Source: CAD feature listing. Evaluate the final solid. Frame: model axes, mm. Face numbers are marked on the shaded views. A direction names the side the tool comes from. Give positions to 0.01 mm unless a question says otherwise; leave off trailing zeros. Loops run counter-clockwise (first coordinate to the right, second up) from the corner with the lowest first, then second, coordinate; pieces in that order, holes last. Notation, with made-up numbers: (75, 40.5) - (82, 40.5) arc R30 ccw to (82, 77.5) - close; hole circle Ø10 at (78.25, 2). An arc over 180 degrees is marked (long way). Write each question's results on one line, items separated by ' | '. Start each with the question number.
(1) Contact query for flat-ended pins moving along their axis: pin 1 (2 mm diameter, centred on x = -11, z = -7.5, fed in from -Y); pin 2 (1.2 mm diameter, centred on y = -0.5, z = 0.5, fed in from -X); pin 3 (3 mm diameter, centred on x = 10.5, z = -3.5, fed in from +Y). Output: stop coordinate, or through.
(2) Material intervals for line 1 along Z through (x, y) = (-11.75, 0.3); line 2 along Z through (x, y) = (-8.25, -0.75); line 3 along X through (y, z) = (-0.1, -2.5), sorted ascending. Write a range as [from, to].
(3) Cut plane A-A on y = -0.8. Return the cut outline in (x, z).
(4) Reachability of the marked faces 1 and 2 from +Z, -Z, +X, -X, +Y, -Y: full face, straight path, thin tool, end or side. Return the list, or none.
Autodesk Inventor part; units mm, degrees
ref_plane "YZ Plane" through (0, 0, 0) normal (1, 0, 0) x (0, 1, 0)
ref_plane "XZ Plane" through (0, 0, 0) normal (0, 1, 0) x (-1, 0, 0)
ref_plane "XY Plane" through (0, 0, 0) normal (0, 0, 1) x (1, 0, 0)
sketch "Sketch1" plane through (0, 0, 0) normal (1, 0, 0) x (0, 1, 0)
  circle A0 centre (0, 0) radius 1.25
  dimension "d0" = 2.5
sketch "Sketch2" plane through (0, 0, 0) normal (0, 1, 0) x (-1, 0, 0)
  line L0 (0, -14.9286) -> (0, 5.5714)
  arc A0 (13.2647, -3.5588) -> (11, 0) centre (11, -2.5) ccw
  arc A1 (-11, 0) -> (-13.2647, -3.5588) centre (-11, -2.5) ccw
  line L1 (11, 0) -> (-11, 0)
  arc A2 (-13.2647, -3.5588) -> (13.2647, -3.5588) centre (0, 2.6429) ccw
  point P0 (0, 0)
  dimension "d4" = 5
  dimension "d5" = 27
  dimension "d6" = 12
sweep "Sweep1" add profiles "Sketch1" path "Sketch2" path curves L1 A1 A2 A0
sketch "Sketch3" plane through (0, 0, 0) normal (0, 1, 0) x (-1, 0, 0)
  line L0 (5, -1.25) -> (-5, -1.25)
  line L1 (-5, -1.25) -> (-5, 1.25)
  line L2 (-5, 1.25) -> (5, 1.25)
  line L3 (5, 1.25) -> (5, -1.25)
  line L4 (11, 1.25) -> (-11, 1.25)
  line L5 (11, -1.25) -> (-11, -1.25)
  point P0 (0, 0)
  point P1 (0, 1.25)
  dimension "d8" = 10
extrude "Extrusion1" cut sketch "Sketch3" along normal through all both and the other way through all
properties part number "Thumb Screw Handle" material "Steel, Mild"
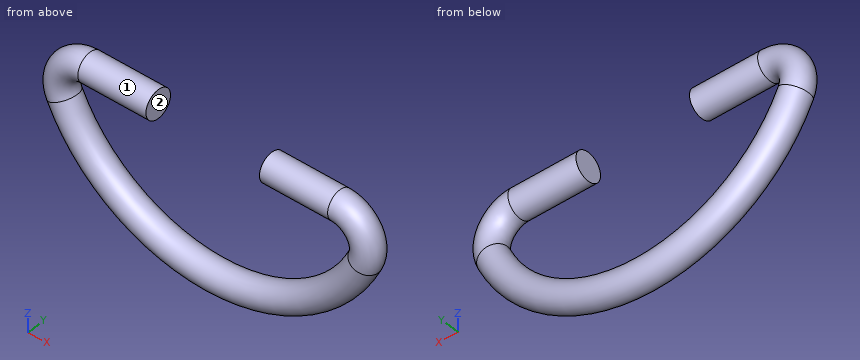
Ans:
1) pin 1: y = -1.25 | pin 2: x = -13.8 | pin 3: y = 0.78
2) line 1: [-8, -3.86], [-1.45, 1.14] | line 2: [-10.65, -8.22], [-1, 1] | line 3: [-14.75, -12.25], [12.25, 14.75]
3) outline: (-14.13, -3.97) arc R15.6 ccw to (14.13, -3.97) arc R3.46 ccw to (11, 0.96) - (5, 0.96) - (5, -0.96) - (11, -0.96) arc R1.54 cw to (12.39, -3.15) arc R13.68 cw to (-12.39, -3.15) arc R1.54 cw to (-11, -0.96) - (-5, -0.96) - (-5, 0.96) - (-11, 0.96) arc R3.46 ccw to start
4) face 1: none | face 2: +Z, +Y, -Y
